Verification items for the finished model (mm, model axes). A direction names the side the tool comes from. Give positions to 0.01 mm unless a question says otherwise; leave off trailing zeros. Write each loop counter-clockwise with the first axis right and the second up, starting at its lowest first coordinate (ties: lowest second). Pieces come first, ordered by that corner, then holes. Notation, with made-up numbers: (17, -35.75) -> (38, -35.75) arc R15 ccw to (38, -11.75) -> close; hole circle Ø9 at (-28, 70). An arc over 180 degrees is marked (long way). Use CSV: the item, a comma, the result in double quotes. Start each with the question number.
```python
from build123d import *

# Parameters (mm, degrees)
F1_DEPTH  = 3
F2_R      = 10
F3_DEPTH  = 150
F4_W      = 4
F4_H      = 47.7245901334
F5_DEPTH  = 146
F7_DEPTH  = 146
F9_DEPTH  = 146
F11_DEPTH = 4
F13_DEPTH = 4
F15_DEPTH = 4
F16_R     = 10
F17_DEPTH = 150
F18_R     = 8
F19_DEPTH = 135
F20_R     = 7.75
F21_DEPTH = 20
F22_SIZE2 = 5.6712818196
F22_SIZE  = 1
F23_R     = 5
F24_DEPTH = 30
F25_R     = 7.75
F26_DEPTH = 20
F27_SIZE2 = 5.6712818196
F27_SIZE  = 1
F28_R     = 5
F29_DEPTH = 30
F30_R     = 7.75
F31_DEPTH = 20
F32_SIZE2 = 5.6712818196
F32_SIZE  = 1
F33_R     = 5
F34_DEPTH = 30
F35_R     = 10
F35_R_2   = 7.75
F36_DEPTH = 150
F37_R     = 10
F37_R_2   = 7.75
F38_DEPTH = 150


# Not quite as in the source:
# - a feature names something its author has since deleted; it is built from what else it names


with BuildPart() as f1:
    # F0 (on Top) → F1 (new body)
    with BuildSketch(Plane.XY):
        Polygon((63.3012701892, -25), (-10, 17.3205080757), (-10, -67.3205080757), align=None)
        Polygon((0, -50), (0, 0), (43.3012701892, -25), align=None, mode=Mode.SUBTRACT)
    extrude(amount=F1_DEPTH)

    # F2 (on face) → F3 (join)
    with BuildSketch(Plane.XY.offset(3)):
        with Locations((-5, 8.6602540378)):
            Circle(F2_R)
        with Locations((53.3012701892, -25)):
            Circle(F2_R)
        with Locations((-5, -58.6602540378)):
            Circle(F2_R)
    extrude(amount=-F3_DEPTH)

    # F4 (on face) → F5 (join)
    with BuildSketch(Plane(origin=(0, 0, 0), x_dir=(1, 0, 0), z_dir=(0, 0, -1))):
        with Locations((-5, 25)):
            Rectangle(F4_W, F4_H)
    extrude(amount=F5_DEPTH)

    # F6 (on face) → F7 (join)
    with BuildSketch(Plane(origin=(0, 0, 0), x_dir=(1, 0, 0), z_dir=(0, 0, -1))):
        Polygon((4.4852813742, -5.4933253598), (45.815988815, 18.3689697069), (43.815988815, 21.833071322), (2.4852813742, -2.0292237447), align=None)
    extrude(amount=F7_DEPTH)

    # F8 (on face) → F9 (join)
    with BuildSketch(Plane(origin=(0, 0, 0), x_dir=(1, 0, 0), z_dir=(0, 0, -1))):
        Polygon((43.815988815, 28.166928678), (45.815988815, 31.6310302931), (4.4852813742, 55.4933253598), (2.4852813742, 52.0292237447), align=None)
    extrude(amount=F9_DEPTH)

    # F10 (on face) → F11 (cut, through all)
    with BuildSketch(Plane(origin=(-7, 0, 0), x_dir=(0, -1, 0), z_dir=(-1, 0, 0))):
        Polygon((48.8622950667, -76), (1.1377049333, -146), (48.8622950667, -146), align=None)
        Polygon((48.8622950667, -70), (48.8622950667, 0), (1.1377049333, 0), align=None)
        Polygon((1.1377049333, -5.3256151295), (1.1377049333, -140.6743848705), (47.2767375115, -73), align=None)
    extrude(amount=-F11_DEPTH, mode=Mode.SUBTRACT)

    # F12 (on face) → F13 (cut, through all)
    with BuildSketch(Plane(origin=(3.5, 6.0621778265, 0), x_dir=(-0.8660254038, 0.5, 0), z_dir=(0.5, 0.8660254038, 0))):
        Polygon((-1.1377049333, -76), (-48.8622950667, -146), (-1.1377049333, -146), align=None)
        Polygon((-1.1377049333, -70), (-1.1377049333, 0), (-48.8622950667, 0), align=None)
        Polygon((-48.8622950667, -5.3256151295), (-48.8622950667, -140.6743848705), (-2.7232624885, -73), align=None)
    extrude(amount=-F13_DEPTH, mode=Mode.SUBTRACT)

    # F14 (on face) → F15 (cut, through all)
    with BuildSketch(Plane(origin=(25.1506350946, -43.5621778265, 0), x_dir=(0.8660254038, 0.5, 0), z_dir=(0.5, -0.8660254038, 0))):
        Polygon((23.8622950667, -76), (-23.8622950667, -146), (23.8622950667, -146), align=None)
        Polygon((23.8622950667, -70), (23.8622950667, 0), (-23.8622950667, 0), align=None)
        Polygon((-23.8622950667, -5.3256151295), (-23.8622950667, -140.6743848705), (22.2767375115, -73), align=None)
    extrude(amount=-F15_DEPTH, mode=Mode.SUBTRACT)

    # F16 (on face) → F17 (join)
    with BuildSketch(Plane(origin=(0, 0, -147), x_dir=(1, 0, 0), z_dir=(0, 0, -1))):
        with Locations((-5, 58.6602540378)):
            Circle(F16_R)
    extrude(amount=-F17_DEPTH)

    # F18 (on face) → F19 (cut)
    with BuildSketch(Plane.XY.offset(3)):
        with Locations((-5, 8.6602540378)):
            Circle(F18_R)
        with Locations((53.3012701892, -25)):
            Circle(F18_R)
        with Locations((-5, -58.6602540378)):
            Circle(F18_R)
    extrude(amount=-F19_DEPTH, mode=Mode.SUBTRACT)

    # F20 (on face) → F21 (join)
    with BuildSketch(Plane(origin=(0, 0, -147), x_dir=(1, 0, 0), z_dir=(0, 0, -1))):
        with Locations((-5, 58.6602540378)):
            Circle(F20_R)
    extrude(amount=F21_DEPTH)

    # F22
    f22_edges = [f1.edges().sort_by_distance(p)[0] for p in [
        (-12.75, -58.660254, -167),
    ]]
    f22_side = f1.faces().sort_by_distance((-5, -58.660254, -167))[0]
    chamfer(f22_edges, length=F22_SIZE, length2=F22_SIZE2, reference=f22_side)

    # F23 (on face) → F24 (cut)
    with BuildSketch(Plane.XY.offset(-132)):
        with Locations((-5, -58.6602540378)):
            Circle(F23_R)
    extrude(amount=-F24_DEPTH, mode=Mode.SUBTRACT)

    # F25 (on face) → F26 (join)
    with BuildSketch(Plane(origin=(0, 0, -147), x_dir=(1, 0, 0), z_dir=(0, 0, -1))):
        with Locations((53.3012701892, 25)):
            Circle(F25_R)
    extrude(amount=F26_DEPTH)

    # F27
    f27_edges = [f1.edges().sort_by_distance(p)[0] for p in [
        (45.55127, -25, -167),
    ]]
    f27_side = f1.faces().sort_by_distance((53.30127, -25, -167))[0]
    chamfer(f27_edges, length=F27_SIZE, length2=F27_SIZE2, reference=f27_side)

    # F28 (on face) → F29 (cut)
    with BuildSketch(Plane.XY.offset(-132)):
        with Locations((53.3012701892, -25)):
            Circle(F28_R)
    extrude(amount=-F29_DEPTH, mode=Mode.SUBTRACT)

    # F30 (on face) → F31 (join)
    with BuildSketch(Plane(origin=(0, 0, -147), x_dir=(1, 0, 0), z_dir=(0, 0, -1))):
        with Locations((-5, -8.6602540378)):
            Circle(F30_R)
    extrude(amount=F31_DEPTH)

    # F32
    f32_edges = [f1.edges().sort_by_distance(p)[0] for p in [
        (-12.75, 8.660254, -167),
    ]]
    f32_side = f1.faces().sort_by_distance((-5, 8.660254, -167))[0]
    chamfer(f32_edges, length=F32_SIZE, length2=F32_SIZE2, reference=f32_side)

    # F33 (on face) → F34 (cut)
    with BuildSketch(Plane.XY.offset(-132)):
        with Locations((-5, 8.6602540378)):
            Circle(F33_R)
    extrude(amount=-F34_DEPTH, mode=Mode.SUBTRACT)

    # F35 (on face) → F36 (join)
    with BuildSketch(Plane(origin=(0, 0, -147), x_dir=(1, 0, 0), z_dir=(0, 0, -1))):
        with Locations((-5, -8.6602540378)):
            Circle(F35_R)
        with Locations((-5, -8.6602540378)):
            Circle(F35_R_2, mode=Mode.SUBTRACT)
    extrude(amount=-F36_DEPTH)

    # F37 (on face) → F38 (join)
    with BuildSketch(Plane(origin=(0, 0, -147), x_dir=(1, 0, 0), z_dir=(0, 0, -1))):
        with Locations((53.3012701892, 25)):
            Circle(F37_R)
        with Locations((53.3012701892, 25)):
            Circle(F37_R_2, mode=Mode.SUBTRACT)
    extrude(amount=-F38_DEPTH)


solid = f1.part
```
(1) Section check D-D on x = -5. Give the number of separate pieces and of enclosed holes in the cut face, then the cut area to 3 significant figures.
(2) Section check B-B on x = 8. Record the cut outline in (y, z), then the cut area to 3 significant figures.
(3) Go/stop test with flat-tipped pins: pin 1 (1.5 mm diameter, centred on y = -22, z = 2, fed in from -X); pin 2 (8 mm diameter, centred on x = 42, z = -91.5, fed in from +Y); pin 3 (3 mm diameter, centred on x = -5, y = 8.5, fed in from +Z); pin 4 (4 mm diameter, centred on x = 19, y = -14, fed in from -Z). Record where each tip stops, or that it passes through.
(4) Draft check along Z on faces 6 (the face through (-5.028, -23.884, -107.311)), 7 (the face through (-1.424, 15.536, -65.445)), 8 (the face through (23.875, -7.979, -110.51)). Enter one of: released by +Z, released by -Z, zero draft, split by the parting line, or undercut.
(5) Section check C-C on y = -10. Record the cut outline in (x, z).
(6) Thickness scan on line 1 (Y direction, x = -5, z = -93); line 2 (Z direction, x = 40, y = -30.5); line 3 (Y direction, x = -5, z = -41). Record the ranges inside material, lowest first. Write a range as from..to.
(7) Set-up check for faces 1 (the face through (-6.7, -51.1, -154.1)), 2 (the face through (-5, -25, -35)), 3 (the face through (-7, -41, -83)), 4 (the face through (25.13, -8.7, -107.31)), 5 (the face through (-5, -59, -162)): record each of +Z, -Z, +X, -X, +Y, -Y from which the full face is reachable in a straight line by a thin tool's end or side.
(8) Section check A-A on z = -150.5. Record the cut outline in (x, y), then the cut area to 3 significant figures.
Data:
1,separate pieces,"1"
1,enclosed holes,"2"
1,area,"2,400 mm2"
2,outline,"(-56.93, 0) -> (-45.38, 0) -> (-45.38, 3) -> (-56.93, 3) -> close; (-53.46, -140.05) -> (-48.85, -136.66) -> (-48.85, -131.33) -> (-53.46, -134.72) -> close; (-53.46, -11.28) -> (-48.85, -14.67) -> (-48.85, -9.34) -> (-53.46, -5.95) -> close; (-4.62, 0) -> (6.93, 0) -> (6.93, 3) -> (-4.62, 3) -> close; (-1.15, -85.34) -> (3.46, -81.95) -> (3.46, -76.63) -> (-1.15, -80.01) -> close; (-1.15, -65.99) -> (3.46, -69.37) -> (3.46, -64.05) -> (-1.15, -60.66) -> close"
2,area,"168 mm2"
3,pin 1,"stops at x = -10"
3,pin 2,"stops at y = -18.17"
3,pin 3,"stops at z = -162"
3,pin 4,"passes through"
4,face 6,"undercut"
4,face 7,"zero draft"
4,face 8,"released by -Z"
5,outline,"(-10, 0) -> (0, 0) -> (0, 3) -> (-10, 3) -> close; (-7, -133) -> (-3, -133) -> (-3, -127.68) -> (-7, -127.68) -> close; (-7, -18.32) -> (-3, -18.32) -> (-3, -13) -> (-7, -13) -> close; (17.32, 0) -> (37.32, 0) -> (37.32, 3) -> (17.32, 3) -> close; (23.32, -111.29) -> (31.32, -121.45) -> (31.32, -116.12) -> (23.32, -105.96) -> close; (23.32, -40.04) -> (31.32, -29.88) -> (31.32, -24.55) -> (23.32, -34.71) -> close"
6,line 1,"y = -68.66..-66.66, -50.66..-48.66, -37.27..-33.64, -1.34..0.91, 16.41..18.66"
6,line 2,"z = -82.56..-77.23, -68.77..-63.44, 0..3"
6,line 3,"y = -68.66..-66.66, -50.66..-48.66, -29.09..-25.46, -1.34..0.91, 16.41..18.66"
7,face 1,"-Z"
7,face 2,"-X"
7,face 3,"-Z, -X"
7,face 4,"none"
7,face 5,"+Z"
8,outline,"circle Ø15.5 at (-5, -58.66); circle Ø15.5 at (-5, 8.66); circle Ø15.5 at (53.3, -25); hole circle Ø10 at (-5, -58.66); hole circle Ø10 at (-5, 8.66); hole circle Ø10 at (53.3, -25)"
8,area,"330 mm2"
